Solid Edge part; units mm, degrees
sketch "Sketch1" plane through (0, 0, 0) normal (0, 1, 0) x (-1, 0, 0)
  line L0 (0, 31.3673) -> (9.3273, 15.6836)
  line L1 (9.3273, 15.6836) -> (16.9273, 15.6836)
  line L2 (16.9273, 15.6836) -> (16.9273, 0)
  line L3 (0, 0) -> (16.9273, 0)
  line L4 (-16.9273, 0) -> (0, 0)
  line L5 (-16.9273, 15.6836) -> (-16.9273, 0)
  line L6 (-9.3273, 15.6836) -> (-16.9273, 15.6836)
  line L7 (0, 31.3673) -> (-9.3273, 15.6836)
extrude "Protrusion1" add sketch "Sketch1" against normal blind 18.4227
sketch "Sketch2" plane through (-13.1273, -9.2114, 15.6836) normal (0, 0, 1) x (-1, 0, 0)
  line L0 (-3.8, -11.3294) -> (-22.4545, -11.3294)
  line L1 (-22.4545, -11.3294) -> (-22.4545, -7.0933)
  line L2 (-22.4545, -7.0933) -> (-3.8, -7.0933)
  line L3 (-3.8, -7.0933) -> (-3.8, -11.3294)
extrude "ExtrudedCutout_1" cut sketch "Sketch2" along normal blind 17.7941
sketch "Sketch3" plane through (0, -18.4227, 15.6836) normal (0, -1, 0) x (1, 0, 0)
  line L0 (9.3273, 16.873) -> (-9.3273, 16.873)
  line L1 (-9.3273, 16.873) -> (-9.3273, 0)
  line L2 (-9.3273, 0) -> (0, 0)
  line L3 (0, 0) -> (9.3273, 0)
  line L4 (9.3273, 0) -> (9.3273, 16.873)
extrude "ExtrudedCutout_2" cut sketch "Sketch3" against normal blind 8.0843
sketch "Sketch4" plane through (0, -18.4227, 7.8418) normal (0, -1, 0) x (1, 0, 0)
  line L0 (-4.6636, 26.1326) -> (4.6636, 26.1326)
  line L1 (4.6636, 7.8418) -> (4.6636, 26.1326)
  line L2 (4.6636, 7.8418) -> (4.6636, -0.7224)
  line L3 (4.6636, -0.7224) -> (0, -0.7224)
  line L4 (-4.6636, -0.7224) -> (0, -0.7224)
  line L5 (-4.6636, 7.8418) -> (-4.6636, -0.7224)
  line L6 (-4.6636, 7.8418) -> (-4.6636, 26.1326)
extrude "ExtrudedCutout_4" cut sketch "Sketch4" against normal blind 11.3261
Input: part model. Units: mm. Frame: model coordinates. A direction names the side the tool comes from. Coordinates: 2 decimals unless noted, no trailing zeros. Write each loop counter-clockwise with the first axis right and the second up, starting at its lowest first coordinate (ties: lowest second). Pieces come first, ordered by that corner, then holes. Notation, with made-up numbers: M 26.5,80 L 54.5,80 A7 cw 54.5,87 Z; hole C -10.75,-26.75 d1. An arc over 180 degrees is marked long. Answer as a JSON object with one key per item and string values. Group by question number.
(1) Section C-C on x = 6. Output: boundary loops of the cut face in (y, z).
(2) Mould query, pull axis X, two halves, no side actions, for faces 4 (the face through (-16.927, -9, 8)), 5 (the face through (4.664, -12, 14)), 6 (the face through (0, -2.118, 22)). Classes: pulls with the +X half, pulls with the -X half, needs draft (parallel to the pull), parting line crosses it, or undercut.
(3) Ray query, line 1 along X through (y, z) = (-7.5, 7.5); line 2 along Y through (x, z) = (-0.5, 21.5); line 3 along Y through (x, z) = (8, 16.5). Return the intervals inside material, ascending. Write a range as [from, to].
(4) Section B-B on z = 13. Output: boundary loops of the cut face in (x, y).
(5) Contact query for flat-ended pins moving along their axis: P1, Ø6, axis at y = -11, z = 16.5, coming from the +X side; P2, Ø3, axis at x = -12, y = -7, coming from the +Z side; P3, Ø7.5, axis at x = -0.5, z = 15, coming from the -Y side; P4, Ø4.5, axis at x = -0.5, y = -15.5, coming from the +Z side. Output: stop coordinate, or through.
(6) Section D-D on y = -8.5. Output: boundary loops of the cut face in (x, z).
(7) Set-up query: faces 1 (the face through (6, -10.338, 18)), 2 (the face through (-4.664, -12, 14)), 3 (the face through (12, -9, 15.684)). Return all of +Z, -Z, +X, -X, +Y, -Y with unobstructed straight access to the full face (end or side cutting, diameter ignored); none if empty.
Result set:
{
 "1": {"outline": "M -18.42,0 L 0,0 L 0,15.68 L -2.12,15.68 L -2.12,21.28 L -10.34,21.28 L -10.34,15.68 L -18.42,15.68 Z"},
 "2": {"face 4": "pulls with the -X half", "face 5": "undercut", "face 6": "needs draft"},
 "3": {"line 1": "x = [-16.93, -4.66], [4.66, 16.93]", "line 2": "y = [-7.1, -2.12]", "line 3": "y = [-10.34, -2.12]"},
 "4": {"outline": "M -16.93,-18.42 L -4.66,-18.42 L -4.66,-7.1 L 4.66,-7.1 L 4.66,-18.42 L 16.93,-18.42 L 16.93,0 L -16.93,0 Z"},
 "5": {"P1": "stops at x = 16.93", "P2": "stops at z = 15.68", "P3": "stops at y = -7.1", "P4": "stops at z = 7.12"},
 "6": {"outline": "M -16.93,0 L 16.93,0 L 16.93,15.68 L 9.33,15.68 L 4.66,23.53 L 4.66,7.12 L -4.66,7.12 L -4.66,23.53 L -9.33,15.68 L -16.93,15.68 Z"},
 "7": {"face 1": "+Z, +X, -X, -Y", "face 2": "+Z, -Y", "face 3": "+Z, +X, -Y"}
}
